Autodesk Fusion 360 part; units mm, degrees
sketch "Sketch1" plane through (0, 0, 0) normal (0, 0, 1) x (1, 0, 0)
  circle A0 centre (0, 0) radius 3.6
  dimension "d1" = 7.2
extrude "Extrude1" add sketch "Sketch1" along normal blind 55
sketch "Sketch2" plane through (0, 0, 55) normal (0, 0, 1) x (-1, 0, 0)
  circle A0 centre (0, 0) radius 3.6
  circle A1 centre (0, 0) radius 2
  dimension "d4" = 4
extrude "Extrude2" cut sketch "Sketch2" against normal blind 6.7 contours A1
sketch "Sketch3" plane through (0, 0, 0) normal (0, 0, -1) x (1, 0, 0)
  circle A0 centre (0, 0) radius 3.6
  circle A1 centre (0, 0) radius 2
  dimension "d7" = 4
extrude "Extrude3" cut sketch "Sketch3" against normal blind 6.7 contours A1
CAD build for the part. Positions are in the model's coordinates, mm. A direction names the side the tool comes from. Give positions to 0.01 mm unless a question says otherwise; leave off trailing zeros. Order: outer loops, then holes, each group sorted by start corner. A loop starts at its lowest first (then second) coordinate and runs counter-clockwise, first axis right, second up. Notation, with made-up numbers: M -30.5,18.25 L -18.5,18.25 A23 cw -18.5,27.25 Z; hole C 13.25,-35.5 d9. An arc over 180 degrees is marked long. Put each result on its own line as item: value. Start each with the question number.
(1) Saw through at A-A, the plane y = 0. Write the cut outline in (x, z), then the cut area to 3 significant figures.
(2) Which spindle directions (+Z, -Z, +X, -X, +Y, -Y) get a long thin tool onto all of the face, cutting with end or side? Do faces 1 (the flat face through (0, 0, 6.7)), 2 (the flat face through (2, -2, 55)). Say none if no direction does.
(3) Mould opens along Y. For faces 3 (the flat face through (2, -2, 0)), 4 (the flat face through (0, 0, 48.3)), 5 (the cylindrical face through (0, 2, 52)), 6 (the cylindrical face through (3.434, -1.081, 27.115)) say: +Y half, -Y half, draft (parallel to the pull), parting line (faces both ways), or undercut.
(4) Drill centre lines: line 1 along Y through (x, z) = (0, 51.5); line 2 along Y through (x, z) = (3, 22); line 3 along Z through (x, y) = (-1.75, -0.5). Where is each one in solid material? Low to high.
(5) Flat gauge pins, fed straight in: pin 1 Ø3.5 at (x, y) = (0, 0) entering from +Z; pin 2 Ø1.5 at (x, z) = (2.5, 41) entering from -Y. Where does each tip first touch, or does it go through?
(6) Saw through at D-D, the plane z = 39. Write the cut outline in (x, y), then the cut area to 3 significant figures.
(7) Saw through at C-C, the plane z = 50.5. Write the cut outline in (x, y), then the cut area to 3 significant figures.
Check result:
1. outline: M -3.6,0 L -2,0 L -2,6.7 L 2,6.7 L 2,0 L 3.6,0 L 3.6,55 L 2,55 L 2,48.3 L -2,48.3 L -2,55 L -3.6,55 Z
1. area: 342 mm2
2. face 1: -Z
2. face 2: +Z, +X, -X, +Y, -Y
3. face 3: draft
3. face 4: undercut
3. face 5: undercut
3. face 6: parting line
4. line 1: y = -3.6 to -2, 2 to 3.6
4. line 2: y = -1.99 to 1.99
4. line 3: z = 6.7 to 48.3
5. pin 1: stops at z = 48.3
5. pin 2: stops at y = -3.15
6. outline: C 0,0 d7.2
6. area: 40.7 mm2
7. outline: C 0,0 d7.2; hole C 0,0 d4
7. area: 28.1 mm2
